Can you work these out from the model? Positions are in its coordinate system, mm. Round coordinates to 2 decimals unless told otherwise and drop trailing zeros. Order: outer loops, then holes, each group sorted by start corner. A loop starts at its lowest first (then second) coordinate and runs counter-clockwise, first axis right, second up.
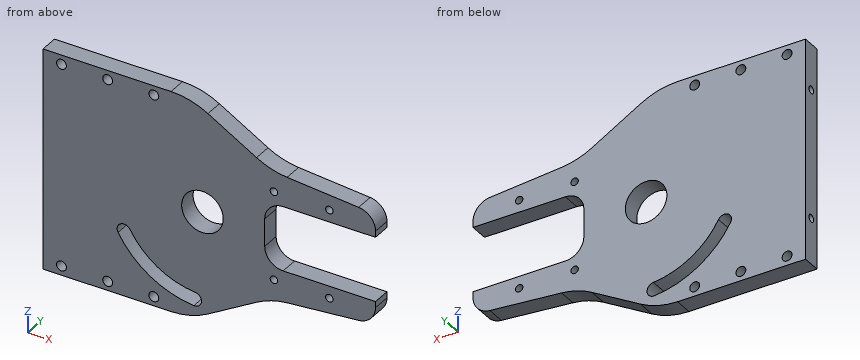
from build123d import *

# Parameters (mm, degrees)
SKETCH2_W                       = 228.6
SKETCH2_H                       = 152.4
BOSS_EXTRUDE1_DEPTH             = 12.7
SKETCH4_W                       = 76.2
SKETCH4_H                       = 44.45
CUT_EXTRUDE1_DEPTH              = 138.957312238
SKETCH5_R                       = 14.2875
CUT_EXTRUDE2_DEPTH              = 138.957312238
CUT_EXTRUDE4_DEPTH              = 138.957312238
TAP_DRILL_FOR_1_4_20_TAP2_D     = 5.1054
FILLET1_R                       = 12.7
TAP_DRILL_FOR_1_4_20_TAP1_D     = 5.1054
TAP_DRILL_FOR_1_4_20_TAP1_DEPTH = 12.7
TAP_DRILL_FOR_1_4_20_TAP1_TIP   = 1.533816902
SKETCH16_W                      = 101.6
SKETCH16_H                      = 12.7
BOSS_EXTRUDE2_DEPTH             = 26.924
BOSS_EXTRUDE3_DEPTH             = 12.7
F_1_4_CLEARANCE_HOLE2_D         = 6.7564
FILLET3_R                       = 50.8
CUT_EXTRUDE5_DEPTH              = 12.7


with BuildPart() as part:
    # Sketch2 → Boss-Extrude1 (new body)
    with BuildSketch(Plane(origin=(0, 0, 0), x_dir=(1, 0, 0), z_dir=(0, 1, 0))):
        Rectangle(SKETCH2_W, SKETCH2_H)
    extrude(amount=-BOSS_EXTRUDE1_DEPTH)

    # Sketch4 → Cut-Extrude1 (cut, through all)
    with BuildSketch(Plane(origin=(0, 0, 0), x_dir=(1, 0, 0), z_dir=(0, 1, 0))):
        with Locations((76.2, 0)):
            Rectangle(SKETCH4_W, SKETCH4_H)
    extrude(amount=-CUT_EXTRUDE1_DEPTH, mode=Mode.SUBTRACT)

    # Sketch5 → Cut-Extrude2 (cut, through all)
    with BuildSketch(Plane(origin=(0, 0, 0), x_dir=(1, 0, 0), z_dir=(0, 1, 0))):
        with Locations(Location((-4.700997292, 0, 0), (0, 0, 270))):
            Circle(SKETCH5_R)
    extrude(amount=-CUT_EXTRUDE2_DEPTH, mode=Mode.SUBTRACT)

    # Sketch8 → Cut-Extrude4 (cut, through all)
    with BuildSketch(Plane(origin=(0, 0, 0), x_dir=(1, 0, 0), z_dir=(0, 1, 0))):
        Polygon((114.3, -38.1), (-12.7, -49.211060268), (-114.3, -49.211060268), (-114.3, -76.2), (114.3, -76.2), align=None)
    cut_extrude4 = extrude(amount=-CUT_EXTRUDE4_DEPTH, mode=Mode.SUBTRACT)

    # Tap Drill for 1/4-20 Tap2 (through all)
    with Locations(Plane(origin=(0, 0, 0), x_dir=(1, 0, 0), z_dir=(0, 1, 0))):
        with Locations((82.55, -30.48), (44.45, -30.48)):
            tap_drill_for_1_4_20_tap2 = Hole(TAP_DRILL_FOR_1_4_20_TAP2_D / 2)

    # Mirror1: Cut-Extrude4, Tap Drill for 1/4-20 Tap2 across plane
    add(cut_extrude4.mirror(Plane.XY), mode=Mode.SUBTRACT)
    add(tap_drill_for_1_4_20_tap2.mirror(Plane.XY), mode=Mode.SUBTRACT)

    # Fillet1
    fillet1_edges = [part.edges().sort_by_distance(p)[0] for p in [
        (38.1, -6.35, 22.225),
        (38.1, -6.35, -22.225),
        (114.3, -6.35, 38.1),
        (114.3, -6.35, -38.1),
    ]]
    fillet(fillet1_edges, radius=FILLET1_R)

    # Tap Drill for 1/4-20 Tap1
    with Locations(Plane.ZY.offset(114.3)):
        with Locations((-44.45, -6.35), (44.45, -6.35)):
            Hole(TAP_DRILL_FOR_1_4_20_TAP1_D / 2, depth=TAP_DRILL_FOR_1_4_20_TAP1_DEPTH)
            with Locations((0, 0, -(TAP_DRILL_FOR_1_4_20_TAP1_DEPTH + TAP_DRILL_FOR_1_4_20_TAP1_TIP / 2))):  # 118° drill point
                Cone(0, TAP_DRILL_FOR_1_4_20_TAP1_D / 2, TAP_DRILL_FOR_1_4_20_TAP1_TIP, mode=Mode.SUBTRACT)

    # Sketch16 → Boss-Extrude2 (add)
    with BuildSketch(Plane.XY.offset(49.211060268)):
        with Locations((-63.5, -6.35)):
            Rectangle(SKETCH16_W, SKETCH16_H)
    boss_extrude2 = extrude(amount=BOSS_EXTRUDE2_DEPTH)

    # Sketch17 → Boss-Extrude3 (add)
    with BuildSketch(Plane.XZ.offset(12.7)):
        Polygon((-12.7, 76.135060268), (42.262462232, 44.402467903), (-12.7, 49.211060268), align=None)
    boss_extrude3 = extrude(amount=-BOSS_EXTRUDE3_DEPTH)

    # 1/4 Clearance Hole2 (through all)
    with Locations(Plane(origin=(0, 0, 0), x_dir=(1, 0, 0), z_dir=(0, 1, 0))):
        with Locations((-101.6, -69.785060268), (-69.85, -69.785060268), (-38.1, -69.785060268)):
            f_1_4_clearance_hole2 = Hole(F_1_4_CLEARANCE_HOLE2_D / 2)

    # Mirror2: Boss-Extrude2, Boss-Extrude3, 1/4 Clearance Hole2 across plane
    add(boss_extrude2.mirror(Plane.XY))
    add(boss_extrude3.mirror(Plane.XY))
    add(f_1_4_clearance_hole2.mirror(Plane.XY), mode=Mode.SUBTRACT)

    # Fillet3
    fillet3_edges = [part.edges().sort_by_distance(p)[0] for p in [
        (-12.7, -6.35, 76.135060268),
        (42.262462232, -6.35, 44.402467903),
        (-12.7, -6.35, -76.135060268),
        (42.262462232, -6.35, -44.402467903),
    ]]
    fillet(fillet3_edges, radius=FILLET3_R)

    # Sketch20 → Cut-Extrude5 (cut)
    with BuildSketch(Plane(origin=(0, 0, 0), x_dir=(1, 0, 0), z_dir=(0, 1, 0))):
        with BuildLine():
            ThreePointArc((-10.539781096, 66.737573312), (-40.696044012, 56.500901434), (-62.718206863, 33.49625))
            ThreePointArc((-62.718206863, 33.49625), (-60.975010878, 26.990554014), (-54.469314892, 28.73375))
            ThreePointArc((-54.469314892, 28.73375), (-35.578265243, 48.467597912), (-9.709622646, 57.248818813))
            ThreePointArc((-9.709622646, 57.248818813), (-5.380324622, 62.408275287), (-10.539781096, 66.737573312))
        make_face()
    extrude(amount=-CUT_EXTRUDE5_DEPTH, mode=Mode.SUBTRACT)


solid = part.part
(1) I want a section at C-C, the plane x = -38.1. List the corners of the cut face in (y, z) for me, plus the area to 3 significant figures.
(2) I want a section at D-D, the plane x = 82.55. List the corners of the cut face in (y, z) for me (3 decimals).
(3) I want a section at A-A, the plane z = 0. List the corners of the cut face in (x, y) for me, plus the area to 3 significant figures.
(4) I want a section at B-B, the plane x = -69.85. List the corners of the cut face in (y, z) for me.
(5) I'm going to push flat-ended pins straight in: pin 1 Ø4 at (x, y) = (58.5, -5.5) entering from -Z; pin 2 Ø3 at (y, z) = (-6.35, -44.45) entering from -X; pin 3 Ø6.5 at (x, y) = (71, -8.5) entering from +Z; pin 4 Ø8 at (x, z) = (44.45, 30.48) entering from +Y. Where does each tip first touch, or does it pass through?
(6) Please list where these lines run through material, in increasing order: probe 1 along Z at (x, y) = (-101.6, -6.5); probe 2 along X at (y, z) = (-2.5, -30.48); probe 3 along Z at (x, y) = (82.55, -5.75) (3 decimals).
Ans:
1. outline: (-12.7, -76.14) - (0, -76.14) - (0, -73.16) - (-12.7, -73.16) - close; (-12.7, -66.41) - (0, -66.41) - (0, -58.07) - (-12.7, -58.07) - close; (-12.7, -46.77) - (0, -46.77) - (0, 66.41) - (-12.7, 66.41) - close; (-12.7, 73.16) - (0, 73.16) - (0, 76.14) - (-12.7, 76.14) - close
1. area: 1,620 mm2
2. outline: (-12.7, -40.878) - (0, -40.878) - (0, -33.033) - (-12.7, -33.033) - close; (-12.7, -27.927) - (0, -27.927) - (0, -22.225) - (-12.7, -22.225) - close; (-12.7, 22.225) - (0, 22.225) - (0, 27.927) - (-12.7, 27.927) - close; (-12.7, 33.033) - (0, 33.033) - (0, 40.878) - (-12.7, 40.878) - close
3. outline: (-114.3, -12.7) - (-18.99, -12.7) - (-18.99, 0) - (-114.3, 0) - close; (9.59, -12.7) - (38.1, -12.7) - (38.1, 0) - (9.59, 0) - close
3. area: 1,570 mm2
4. outline: (-12.7, -76.14) - (0, -76.14) - (0, -73.16) - (-12.7, -73.16) - close; (-12.7, -66.41) - (0, -66.41) - (0, 66.41) - (-12.7, 66.41) - close; (-12.7, 73.16) - (0, 73.16) - (0, 76.14) - (-12.7, 76.14) - close
5. pin 1: stops at z = -43.16
5. pin 2: stops at x = -100.97
5. pin 3: stops at z = 42.17
5. pin 4: stops at y = 0
6. probe 1: z = -76.14 to -73.16, -66.41 to -47, -41.9 to 41.9, 47 to 66.41, 73.16 to 76.14
6. probe 2: x = -114.3 to -63.31, -53.42 to 41.9, 47 to 80, 85.1 to 113.65
6. probe 3: z = -40.878 to -33.033, -27.927 to -22.225, 22.225 to 27.927, 33.033 to 40.878
